from build123d import *

# Parameters (mm, degrees)
F0_W      = 125
F0_H      = 20
F1_DEPTH  = 5
F2_W      = 125
F2_H      = 6
F3_DEPTH  = 5
F4_R      = 2.75
F5_DEPTH  = 25
F6_W      = 11.2
F6_H      = 6
F7_DEPTH  = 5
F8_R      = 2.6
F9_DEPTH  = 5
F10_R     = 2.6
F11_DEPTH = 4
F12_R     = 1
F13_SIZE2 = 0.5
F13_SIZE  = 0.2886751346


with BuildPart() as f1:
    # F0 (on Top) → F1 (new body)
    with BuildSketch(Plane.XY):
        with Locations((62.5, 0)):
            Rectangle(F0_W, F0_H)
    extrude(amount=F1_DEPTH)

    # F2 (on face) → F3 (join)
    with BuildSketch(Plane.XY.offset(5)):
        with Locations((62.5, 0)):
            Rectangle(F2_W, F2_H)
    extrude(amount=F3_DEPTH)

    # F4 (on face) → F5 (cut)
    with BuildSketch(Plane.XY.offset(10)):
        with Locations((98, 0)):
            Circle(F4_R)
        with Locations((78, 0)):
            Circle(F4_R)
        with Locations((58, 0)):
            Circle(F4_R)
    extrude(amount=-F5_DEPTH, mode=Mode.SUBTRACT)

    # F6 (on face) → F7 (cut, through all)
    with BuildSketch(Plane.XY.offset(10)):
        with Locations((109.6, 0)):
            Rectangle(F6_W, F6_H)
        with Locations((46.4, 0)):
            Rectangle(F6_W, F6_H)
    extrude(amount=-F7_DEPTH, mode=Mode.SUBTRACT)

    # F8 (on face) → F9 (cut, through all)
    with BuildSketch(Plane.XY.offset(5)):
        with Locations((46.4, 0)):
            Circle(F8_R)
        with Locations((109.6, 0)):
            Circle(F8_R)
    extrude(amount=-F9_DEPTH, mode=Mode.SUBTRACT)

    # F10 (on face) → F11 (join)
    with BuildSketch(Plane(origin=(0, 0, 0), x_dir=(0, -1, 0), z_dir=(-1, 0, 0))):
        Polygon((-10, 25), (-10, 5), (-3, 5), (-3, 10), (3, 10), (3, 5), (10, 5), (10, 25), align=None)
        with Locations((0, 15)):
            Circle(F10_R, mode=Mode.SUBTRACT)
        Polygon((-10, 5), (-10, 0), (10, 0), (10, 5), (3, 5), (3, 10), (-3, 10), (-3, 5), align=None)
    extrude(amount=F11_DEPTH)

    # F12
    f12_edges = [f1.edges().sort_by_distance(p)[0] for p in [
        (-2, -10, 25),
        (-2, 10, 25),
        (60.5, -10, 0),
        (60.5, 10, 0),
    ]]
    fillet(f12_edges, radius=F12_R)

    # F13
    f13_edges = [f1.edges().sort_by_distance(p)[0] for p in [
        (55.25, 0, 0),
        (75.25, 0, 0),
        (95.25, 0, 0),
    ]]
    f13_side = f1.faces().sort_by_distance((-2.697502, 0, 0))[0]
    chamfer(f13_edges, length=F13_SIZE, length2=F13_SIZE2, reference=f13_side)


solid = f1.part
Input: part model. Units: mm. Frame: model coordinates. A direction names the side the tool comes from. Coordinates: 2 decimals unless noted, no trailing zeros. Loops run counter-clockwise (first coordinate to the right, second up) from the corner with the lowest first, then second, coordinate; pieces in that order, holes last. Notation, with made-up numbers: (-20, -19.5) -> (12, -19.5) arc R16 ccw to (12, -5.5) -> close; hole circle Ø9 at (62, 35.25). An arc over 180 degrees is marked (long way). Write each question's results on one line, items separated by ' | '. Start each with the question number.
Q1. Pull-direction query (Z, two-part tool) for faces 1 (the cylindrical face through (-1.97, 0.56, 12.46)), 2 (the cylindrical face through (44.484, 1.757, 2.535)), 3 (the flat face through (83, 0, 10)); classes: released by +Z, released by -Z, zero draft, split by the parting line, or undercut.
Q2. Ray query, line 1 (Y direction, x = 58, z = 8); line 2 (X direction, y = -0.5, z = 8.75); line 3 (Z direction, x = 95, y = -8). Return the intervals inside material, ascending. Write a range as from..to.
Q3. Section A-A, the plane z = 15. Return the cut outline in (x, y).
Q4. Section C-C, the plane z = 3. Return the cut outline in (x, y), plus the area to 3 significant figures.
Q5. Section D-D, the plane y = 0. State how many separate pieces and enclosed holes the cut face has, plus the area to 4 significant figures.
Q6. Pin query (flat end, axial travel): pin 1 (10 mm diameter, centred on x = 48, y = 0, fed in from +Z); pin 2 (2.5 mm diameter, centred on x = 87.5, z = 7.5, fed in from -Y); pin 3 (1.5 mm diameter, centred on x = 72, y = 0.5, fed in from -Z); pin 4 (10 mm diameter, centred on x = 54, z = 11, fed in from +Y). Return the tip coordinate at first contact, or that it passes through.
Q7. Reachability of faces 4 (the flat face through (52, 0, 8)), 5 (the flat face through (120, -3, 7)), 6 (the flat face through (51, 10, 3)), 7 (the flat face through (78, 3, 7)), 8 (the cylindrical face through (55.253, 0.121, 5.316)) from +Z, -Z, +X, -X, +Y, -Y: full face, straight path, thin tool, end or side. Return the list, or none.
Q8. Section B-B, the plane x = 78. Return the cut outline in (y, z), plus the area to 3 significant figures.
Found:
1) face 1: undercut | face 2: zero draft | face 3: released by +Z
2) line 1: -3..-2.75, 2.75..3 | line 2: -4..40.8, 52..55.3, 60.7..75.3, 80.7..95.3, 100.7..104, 115.2..125 | line 3: 0..5
3) outline: (-4, -10) -> (0, -10) -> (0, -2.6) -> (-4, -2.6) -> close; (-4, 2.6) -> (0, 2.6) -> (0, 10) -> (-4, 10) -> close
4) outline: (-4, -10) -> (125, -10) -> (125, 10) -> (-4, 10) -> close; hole circle Ø5.2 at (46.4, 0); hole circle Ø5.5 at (58, 0); hole circle Ø5.5 at (78, 0); hole circle Ø5.5 at (98, 0); hole circle Ø5.2 at (109.6, 0) | area: 2,470 mm2
5) separate pieces: 7 | enclosed holes: 0 | area: 1,000 mm2
6) pin 1: z = 10 | pin 2: y = -3 | pin 3: z = 0 | pin 4: y = 3
7) face 4: +Z, +Y, -Y | face 5: +Z, +X, -Y | face 6: +Z, -Z, +X, -X, +Y | face 7: +Z, +X, +Y | face 8: +Z, -Z
8) outline: (-10, 1) arc R1 ccw to (-9, 0) -> (-3.04, 0) -> (-2.75, 0.5) -> (-2.75, 10) -> (-3, 10) -> (-3, 5) -> (-10, 5) -> close; (2.75, 0.5) -> (3.04, 0) -> (9, 0) arc R1 ccw to (10, 1) -> (10, 5) -> (3, 5) -> (3, 10) -> (2.75, 10) -> close | area: 74.4 mm2
